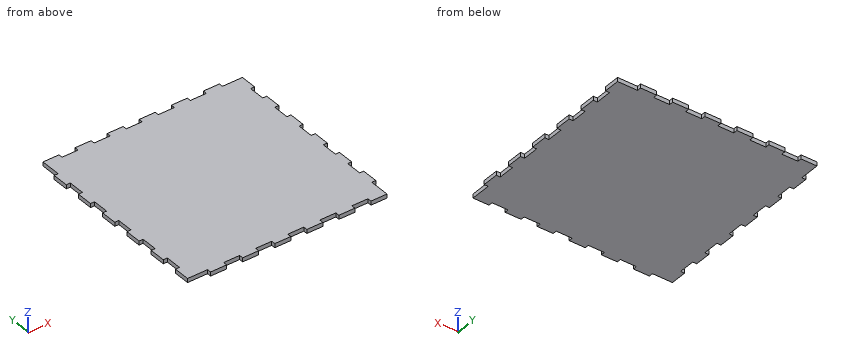
Autodesk Inventor part; units mm, degrees
ref_plane "YZ Plane" through (0, 0, 0) normal (1, 0, 0) x (0, 1, 0)
ref_plane "XZ Plane" through (0, 0, 0) normal (0, 1, 0) x (-1, 0, 0)
ref_plane "XY Plane" through (0, 0, 0) normal (0, 0, 1) x (1, 0, 0)
sketch "Sketch1" plane through (0, 0, 0) normal (0, 0, 1) x (1, 0, 0)
  line L0 (425.9934, 353.49) -> (405.9934, 353.49)
  line L1 (185.9934, 353.49) -> (185.9934, 358.49)
  line L2 (185.9934, 358.49) -> (205.9934, 358.49)
  line L3 (205.9934, 358.49) -> (205.9934, 353.49)
  line L4 (225.9934, 353.49) -> (225.9934, 358.49)
  line L5 (225.9934, 358.49) -> (245.9934, 358.49)
  line L6 (245.9934, 358.49) -> (245.9934, 353.49)
  line L7 (265.9934, 353.49) -> (265.9934, 358.49)
  line L8 (265.9934, 358.49) -> (285.9934, 358.49)
  line L9 (285.9934, 358.49) -> (285.9934, 353.49)
  line L10 (305.9934, 353.49) -> (305.9934, 358.49)
  line L11 (305.9934, 358.49) -> (325.9934, 358.49)
  line L12 (325.9934, 358.49) -> (325.9934, 353.49)
  line L13 (345.9934, 353.49) -> (345.9934, 358.49)
  line L14 (345.9934, 358.49) -> (365.9934, 358.49)
  line L15 (365.9934, 358.49) -> (365.9934, 353.49)
  line L16 (385.9934, 353.49) -> (385.9934, 358.49)
  line L17 (385.9934, 358.49) -> (405.9934, 358.49)
  line L18 (405.9934, 358.49) -> (405.9934, 353.49)
  line L19 (385.9934, 353.49) -> (365.9934, 353.49)
  line L20 (345.9934, 353.49) -> (325.9934, 353.49)
  line L21 (305.9934, 353.49) -> (285.9934, 353.49)
  line L22 (265.9934, 353.49) -> (245.9934, 353.49)
  line L23 (225.9934, 353.49) -> (205.9934, 353.49)
  line L24 (425.9934, 113.49) -> (425.9934, 133.49)
  line L25 (425.9934, 353.49) -> (430.9934, 353.49)
  line L26 (430.9934, 353.49) -> (430.9934, 333.49)
  line L27 (430.9934, 333.49) -> (425.9934, 333.49)
  line L28 (425.9934, 313.49) -> (430.9934, 313.49)
  line L29 (430.9934, 313.49) -> (430.9934, 293.49)
  line L30 (430.9934, 293.49) -> (425.9934, 293.49)
  line L31 (425.9934, 273.49) -> (430.9934, 273.49)
  line L32 (430.9934, 273.49) -> (430.9934, 253.49)
  line L33 (430.9934, 253.49) -> (425.9934, 253.49)
  line L34 (425.9934, 233.49) -> (430.9934, 233.49)
  line L35 (430.9934, 233.49) -> (430.9934, 213.49)
  line L36 (430.9934, 213.49) -> (425.9934, 213.49)
  line L37 (425.9934, 193.49) -> (430.9934, 193.49)
  line L38 (430.9934, 193.49) -> (430.9934, 173.49)
  line L39 (430.9934, 173.49) -> (425.9934, 173.49)
  line L40 (425.9934, 153.49) -> (430.9934, 153.49)
  line L41 (430.9934, 153.49) -> (430.9934, 133.49)
  line L42 (430.9934, 133.49) -> (425.9934, 133.49)
  line L43 (425.9934, 153.49) -> (425.9934, 173.49)
  line L44 (425.9934, 193.49) -> (425.9934, 213.49)
  line L45 (425.9934, 233.49) -> (425.9934, 253.49)
  line L46 (425.9934, 273.49) -> (425.9934, 293.49)
  line L47 (425.9934, 313.49) -> (425.9934, 333.49)
  line L48 (185.9934, 353.49) -> (185.9934, 333.49)
  line L49 (185.9934, 113.49) -> (180.9934, 113.49)
  line L50 (180.9934, 113.49) -> (180.9934, 133.49)
  line L51 (180.9934, 133.49) -> (185.9934, 133.49)
  line L52 (185.9934, 153.49) -> (180.9934, 153.49)
  line L53 (180.9934, 153.49) -> (180.9934, 173.49)
  line L54 (180.9934, 173.49) -> (185.9934, 173.49)
  line L55 (185.9934, 193.49) -> (180.9934, 193.49)
  line L56 (180.9934, 193.49) -> (180.9934, 213.49)
  line L57 (180.9934, 213.49) -> (185.9934, 213.49)
  line L58 (185.9934, 233.49) -> (180.9934, 233.49)
  line L59 (180.9934, 233.49) -> (180.9934, 253.49)
  line L60 (180.9934, 253.49) -> (185.9934, 253.49)
  line L61 (185.9934, 273.49) -> (180.9934, 273.49)
  line L62 (180.9934, 273.49) -> (180.9934, 293.49)
  line L63 (180.9934, 293.49) -> (185.9934, 293.49)
  line L64 (185.9934, 313.49) -> (180.9934, 313.49)
  line L65 (180.9934, 313.49) -> (180.9934, 333.49)
  line L66 (180.9934, 333.49) -> (185.9934, 333.49)
  line L67 (185.9934, 313.49) -> (185.9934, 293.49)
  line L68 (185.9934, 273.49) -> (185.9934, 253.49)
  line L69 (185.9934, 233.49) -> (185.9934, 213.49)
  line L70 (185.9934, 193.49) -> (185.9934, 173.49)
  line L71 (185.9934, 153.49) -> (185.9934, 133.49)
  line L72 (185.9934, 113.49) -> (205.9934, 113.49)
  line L73 (425.9934, 113.49) -> (425.9934, 108.49)
  line L74 (425.9934, 108.49) -> (405.9934, 108.49)
  line L75 (405.9934, 108.49) -> (405.9934, 113.49)
  line L76 (385.9934, 113.49) -> (385.9934, 108.49)
  line L77 (385.9934, 108.49) -> (365.9934, 108.49)
  line L78 (365.9934, 108.49) -> (365.9934, 113.49)
  line L79 (345.9934, 113.49) -> (345.9934, 108.49)
  line L80 (345.9934, 108.49) -> (325.9934, 108.49)
  line L81 (325.9934, 108.49) -> (325.9934, 113.49)
  line L82 (305.9934, 113.49) -> (305.9934, 108.49)
  line L83 (305.9934, 108.49) -> (285.9934, 108.49)
  line L84 (285.9934, 108.49) -> (285.9934, 113.49)
  line L85 (265.9934, 113.49) -> (265.9934, 108.49)
  line L86 (265.9934, 108.49) -> (245.9934, 108.49)
  line L87 (245.9934, 108.49) -> (245.9934, 113.49)
  line L88 (225.9934, 113.49) -> (225.9934, 108.49)
  line L89 (225.9934, 108.49) -> (205.9934, 108.49)
  line L90 (205.9934, 108.49) -> (205.9934, 113.49)
  line L91 (225.9934, 113.49) -> (245.9934, 113.49)
  line L92 (265.9934, 113.49) -> (285.9934, 113.49)
  line L93 (305.9934, 113.49) -> (325.9934, 113.49)
  line L94 (345.9934, 113.49) -> (365.9934, 113.49)
  line L95 (385.9934, 113.49) -> (405.9934, 113.49)
  point P0 (0, 0)
extrude "Extrusion1" add sketch "Sketch1" along normal blind 5
sketch "Sketch2" plane through (0, 0, 5) normal (0, 0, 1) x (1, 0, 0)
  point P0 (0, 0)
properties material "Glass"
Verification items for the finished model (mm, model axes). Give positions to 0.01 mm unless a question says otherwise; leave off trailing zeros. Write each loop counter-clockwise with the first axis right and the second up, starting at its lowest first coordinate (ties: lowest second). Pieces come first, ordered by that corner, then holes.
(1) Cross-section at A-A (x = 361.5). Enter the section's corners in (y, z), plus the area to 4 significant figures.
(2) Material ranges on line 1 (Y direction, x = 194, z = 0.45); line 2 (X direction, y = 162.5, z = 0.6); line 3 (X direction, y = 266, z = 1.1), recorded low to high.
(3) Cross-section at B-B (y = 163). Enter the section's corners in (x, z), plus the area to 4 significant figures.
(4) Gauge pin test, flat ends, axial feed: pin 1 (2.5 mm diameter, centred on y = 299, z = 1.5, fed in from -X); pin 2 (1 mm diameter, centred on y = 283.5, z = 4.5, fed in from +X); pin 3 (1.5 mm diameter, centred on x = 428, z = 1.5, fed in from +Y). Record the tip position at first contact, or that the pin passes through.
Worked out:
1. outline: (113.49, 0) - (358.49, 0) - (358.49, 5) - (113.49, 5) - close
1. area: 1,225 mm2
2. line 1: y = 113.49 to 358.49
2. line 2: x = 180.99 to 425.99
2. line 3: x = 185.99 to 430.99
3. outline: (180.99, 0) - (425.99, 0) - (425.99, 5) - (180.99, 5) - close
3. area: 1,225 mm2
4. pin 1: stops at x = 185.99
4. pin 2: stops at x = 425.99
4. pin 3: stops at y = 353.49
